For this review, take the finished solid that the model builds, in its own axes (mm). Face numbers are marked on the shaded views. A direction names the side the tool comes from. Coordinates: 2 decimals unless noted, no trailing zeros. Loops run counter-clockwise (first coordinate to the right, second up) from the corner with the lowest first, then second, coordinate; pieces in that order, holes last. Notation, with made-up numbers: (15, 62.25) -> (65, 62.25) arc R17 ccw to (65, 89.25) -> close; hole circle Ø6 at (2.25, 35). An arc over 180 degrees is marked (long way). Answer in a Markdown table with one row per item.
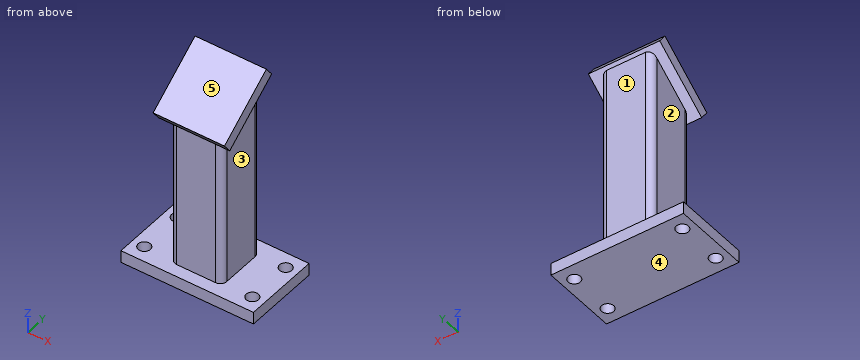
from build123d import *

# Parameters (mm, degrees)
F0_W     = 130
F0_H     = 75
F1_DEPTH = 12
F3_DEPTH = 185
F5_D     = 12
F7_DEPTH = 50.8
F8_W     = 70
F8_H     = 70
F9_DEPTH = 12


with BuildPart() as f1:
    # F0 (on Top) → F1 (new body)
    with BuildSketch(Plane.XY):
        Rectangle(F0_W, F0_H)
    extrude(amount=-F1_DEPTH)

    # F2 (on face) → F3 (join)
    with BuildSketch(Plane.XY):
        with BuildLine():
            Line((-19.05, -25.4), (19.05, -25.4))
            ThreePointArc((19.05, -25.4), (23.540128, -23.540128), (25.4, -19.05))
            Line((25.4, -19.05), (25.4, 19.05))
            ThreePointArc((25.4, 19.05), (23.540128, 23.540128), (19.05, 25.4))
            Line((19.05, 25.4), (-19.05, 25.4))
            ThreePointArc((-19.05, 25.4), (-23.540128, 23.540128), (-25.4, 19.05))
            Line((-25.4, 19.05), (-25.4, -19.05))
            ThreePointArc((-25.4, -19.05), (-23.540128, -23.540128), (-19.05, -25.4))
        make_face()
        with BuildLine():
            Line((-12.7, 19.05), (12.7, 19.05))
            ThreePointArc((12.7, 19.05), (17.190128, 17.190128), (19.05, 12.7))
            Line((19.05, 12.7), (19.05, -12.7))
            ThreePointArc((19.05, -12.7), (17.190128, -17.190128), (12.7, -19.05))
            Line((12.7, -19.05), (-12.7, -19.05))
            ThreePointArc((-12.7, -19.05), (-17.190128, -17.190128), (-19.05, -12.7))
            Line((-19.05, -12.7), (-19.05, 12.7))
            ThreePointArc((-19.05, 12.7), (-17.190128, 17.190128), (-12.7, 19.05))
        make_face(mode=Mode.SUBTRACT)
    extrude(amount=F3_DEPTH)

    # F5 (through all)
    with Locations(Plane.XY):
        with Locations((-53, 22.5), (53, 22.5), (53, -22.5), (-53, -22.5)):
            Hole(F5_D / 2)

    # F6 (on face) → F7 (cut)
    with BuildSketch(Plane.YZ.offset(25.4)):
        Polygon((25.4, 185), (-25.4, 185), (-25.4, 147.956003), align=None)
    extrude(amount=-F7_DEPTH, mode=Mode.SUBTRACT)

    # F8 (on face) → F9 (join)
    with BuildSketch(Plane(origin=(0, -79.254299, 108.684772), x_dir=(1, 0, 0), z_dir=(0, -0.589196, 0.80799))):
        with Locations((0, 98.088232)):
            Rectangle(F8_W, F8_H)
    extrude(amount=F9_DEPTH)


solid = f1.part
Item 1: Take a section at D-D, the plane y = -22.5. State the section outline as (x, z) points.
Worked answers:
| item | result |
|---|---|
| outline | (-65, -12) -> (-59, -12) -> (-59, 0) -> (-65, 0) -> close; (-47, -12) -> (47, -12) -> (47, 0) -> (24.38, 0) -> (24.38, 150.07) -> (35, 150.07) -> (35, 164.92) -> (-35, 164.92) -> (-35, 150.07) -> (-24.38, 150.07) -> (-24.38, 0) -> (-47, 0) -> close; (59, -12) -> (65, -12) -> (65, 0) -> (59, 0) -> close |
Item 2: Insertion check: pin 1 (10 mm diameter, centred on x = 23.5, z = 122.5, fed in from +Y); pin 2 (8 mm diameter, centred on y = 14.5, z = 11.5, fed in from -X); pin 3 (19 mm diameter, centred on x = -2.5, z = 38, fed in from -Y); pin 4 (15.5 mm diameter, centred on x = 53, y = -22.5, fed in from -Z). Each pin has a flat end and moves straight along its axis. Give the tip position at first contact, or say it passes through.
Worked answers:
| item | result |
|---|---|
| pin 1 | y = 25.4 |
| pin 2 | x = -25.4 |
| pin 3 | y = -25.4 |
| pin 4 | z = -12 |
Item 3: Take a section at B-B, the plane z = 75. State the section outline as (x, y) points.
Worked answers:
| item | result |
|---|---|
| outline | (-25.4, -19.05) arc R6.35 ccw to (-19.05, -25.4) -> (19.05, -25.4) arc R6.35 ccw to (25.4, -19.05) -> (25.4, 19.05) arc R6.35 ccw to (19.05, 25.4) -> (-19.05, 25.4) arc R6.35 ccw to (-25.4, 19.05) -> close; hole (-19.05, -12.7) arc R6.35 ccw to (-12.7, -19.05) -> (12.7, -19.05) arc R6.35 ccw to (19.05, -12.7) -> (19.05, 12.7) arc R6.35 ccw to (12.7, 19.05) -> (-12.7, 19.05) arc R6.35 ccw to (-19.05, 12.7) -> close |
Item 4: Take a section at A-A, the plane x = -53. State the section outline as (y, z) points, and give its area (3 significant figures).
Worked answers:
| item | result |
|---|---|
| outline | (-37.5, -12) -> (-28.5, -12) -> (-28.5, 0) -> (-37.5, 0) -> close; (-16.5, -12) -> (16.5, -12) -> (16.5, 0) -> (-16.5, 0) -> close; (28.5, -12) -> (37.5, -12) -> (37.5, 0) -> (28.5, 0) -> close |
| area | 612 mm² |
Item 5: For L1, parallel to X at y = 22, z = -7; L2, parallel to Y at x = -53, z = -8.75; L3, parallel to X at y = 4.5, z = 16.5, list the stretches that pass through material, from the lowest coordinate up.
Worked answers:
| item | result |
|---|---|
| L1 | -65 to -58.98, -47.02 to 47.02, 58.98 to 65 |
| L2 | -37.5 to -28.5, -16.5 to 16.5, 28.5 to 37.5 |
| L3 | -25.4 to -19.05, 19.05 to 25.4 |
Item 6: For the marked faces 1 and 2, list the 3-axis set-ups (+Z, -Z, +X, -X, +Y, -Y) from which the entire face can be reached by the end or side of a thin tool; tool diameter is ignored.
Worked answers:
| item | result |
|---|---|
| face 1 | +X, -X, +Y |
| face 2 | -X, +Y |
Item 7: Take a section at C-C, the plane y = -3.5. State the section outline as (x, z) points.
Worked answers:
| item | result |
|---|---|
| outline | (-65, -12) -> (65, -12) -> (65, 0) -> (25.4, 0) -> (25.4, 163.93) -> (35, 163.93) -> (35, 178.78) -> (-35, 178.78) -> (-35, 163.93) -> (-25.4, 163.93) -> (-25.4, 0) -> (-65, 0) -> close; hole (-19.05, 0) -> (19.05, 0) -> (19.05, 163.93) -> (-19.05, 163.93) -> close |
Item 8: The part is to be moulded in two halves that separate along Z. For the marked faces 3, 4 and 5, say which applies: +Z half, -Z half, draft (parallel to the pull), parting line (faces both ways), or undercut.
Worked answers:
| item | result |
|---|---|
| face 3 | undercut |
| face 4 | -Z half |
| face 5 | +Z half |
